Build history of the part. All positions in model axes, mm. A direction names the side the tool comes from. Round coordinates to 2 decimals unless told otherwise and drop trailing zeros. Write each loop counter-clockwise with the first axis right and the second up, starting at its lowest first coordinate (ties: lowest second). Pieces come first, ordered by that corner, then holes. Notation, with made-up numbers: (-12.75, -32.75) -> (8.25, -32.75) arc R21 ccw to (8.25, -25.75) -> close; hole circle Ø3 at (38.25, 39.25). An arc over 180 degrees is marked (long way). Answer in a Markdown table with one row per item. Add a question column.
from build123d import *

# Parameters (mm, degrees)
SKETCH_1_R      = 2.3
EXTRUDE_1_DEPTH = 10
SKETCH_2_W      = 10
SKETCH_2_H      = 15
EXTRUDE_2_DEPTH = 100
SKETCH_3_R      = 2.3
EXTRUDE_3_DEPTH = 10
CHAMFER_1_SIZE  = 5


with BuildPart() as part:
    # Эскиз1 → Бобышка-Вытянуть1 (new body)
    with BuildSketch(Plane(origin=(0, 116.195974268, 0), x_dir=(1, 0, 0), z_dir=(0, 1, 0))):
        Polygon((-8.441019306, -97.523129836), (-8.441019306, -81.523129836), (-8.441019306, -66.523129836), (1.558980694, -66.523129836), (1.558980694, -112.523129836), (-8.441019306, -112.523129836), align=None)
        with Locations(Location((-3.441019306, -89.187817333, 0), (0, 0, 180))):
            Circle(SKETCH_1_R, mode=Mode.SUBTRACT)
    extrude(amount=EXTRUDE_1_DEPTH)

    # Эскиз2 → Бобышка-Вытянуть2 (add)
    with BuildSketch(Plane(origin=(0, 126.195974268, 0), x_dir=(1, 0, 0), z_dir=(0, 1, 0))):
        with Locations((-3.441019306, -74.023129836)):
            Rectangle(SKETCH_2_W, SKETCH_2_H)
        with Locations((-3.441019306, -105.023129836)):
            Rectangle(SKETCH_2_W, SKETCH_2_H)
    extrude(amount=EXTRUDE_2_DEPTH)

    # Эскиз3 → Бобышка-Вытянуть3 (add)
    with BuildSketch(Plane(origin=(0, 226.195974268, 0), x_dir=(1, 0, 0), z_dir=(0, 1, 0))):
        Polygon((-8.441019306, -66.543886748), (-8.441019306, -112.425486731), (1.558980694, -112.523129836), (1.558980694, -66.523129836), align=None)
        with Locations(Location((-3.441019306, -89.187817333, 0), (0, 0, 180))):
            Circle(SKETCH_3_R, mode=Mode.SUBTRACT)
    extrude(amount=EXTRUDE_3_DEPTH)

    # Фаска1
    # the kernel refuses this chamfer: 5 mm, written as the material it takes off along each edge
    with BuildSketch(Plane(origin=(-8.441019306, 239.054389208, 66.523129836), x_dir=(-0.027495876610586625, 0, 0.9996219169112968), z_dir=(0, -1, 0)), Plane(origin=(-8.441019306, 103.337559328, 112.523129836), x_dir=(-0.027495876610585935, 0, -0.9996219169112968), z_dir=(0, 1, 0))) as chamfer_1_piece_1:
        Polygon((CHAMFER_1_SIZE * 0.999621916911, -CHAMFER_1_SIZE * 0.0274958766106), (-CHAMFER_1_SIZE * 0.0274958766106, -CHAMFER_1_SIZE * 0.999621916911), (0, 0), align=None)
    extrude(amount=135.71682988, mode=Mode.SUBTRACT)


solid = part.part
(1) Probe line 1 along Y through (x, z) = (-5.75, 94); line 2 along Z through (x, y) = (-0.75, 154); line 3 along Z through (x, y) = (-3.5, 149). List the from-to ranges inside material, lowest first.
(2) Mould opens along Y. For faces 3 (the face through (-6, 226.196, 89)), 4 (the face through (-5.976, 175.356, 109.988)), 5 (the face through (0, 236.196, 89)) say: pulls with the +Y half, pulls with the -Y half, needs draft (parallel to the pull), parting line crosses it, or undercut.
(3) Saw through at C-C (x = -7). List the corners of the cut face in (y, z).
(4) Saw through at B-B (z = 84). List the corners of the cut face in (x, y).
(5) Saw through at A-A (y = 212). List the corners of the cut face in (x, z).
(6) Drop flat-ended pins along their axis: P1, Ø6, axis at x = -3.44, z = 89.19, coming from the +Y side; P2, Ø10, axis at y = 199, z = 90.5, coming from the -X side; P3, Ø5, axis at x = -7.5, y = 174.5, coming from the -Z side. Give the stop position or say it passes through.
(7) Which spindle directions (+Z, -Z, +X, -X, +Y, -Y) get a long thin tool onto all of the face, cutting with end or side? Do faces 1 (the face through (-5.98, 177.04, 69.06)), 2 (the face through (-4, 175, 81.523)). Say none if no direction does.
Answer sheet:
| question | item | result |
|---|---|---|
| 1 | line 1 | y = 116.2 to 126.2, 226.2 to 236.2 |
| 1 | line 2 | z = 66.52 to 81.52, 97.52 to 112.52 |
| 1 | line 3 | z = 66.58 to 81.52, 97.52 to 112.46 |
| 2 | face 3 | undercut |
| 2 | face 4 | needs draft |
| 2 | face 5 | pulls with the +Y half |
| 3 | outline | (116.2, 70.08) -> (236.2, 70.08) -> (236.2, 108.96) -> (116.2, 108.96) -> close; hole (126.2, 81.52) -> (226.2, 81.52) -> (226.2, 97.52) -> (126.2, 97.52) -> close |
| 4 | outline | (-8.44, 116.2) -> (1.56, 116.2) -> (1.56, 126.2) -> (-8.44, 126.2) -> close; (-8.44, 226.2) -> (1.56, 226.2) -> (1.56, 236.2) -> (-8.44, 236.2) -> close |
| 5 | outline | (-8.44, 71.52) -> (-3.44, 66.52) -> (1.56, 66.52) -> (1.56, 81.52) -> (-8.44, 81.52) -> close; (-8.44, 97.52) -> (1.56, 97.52) -> (1.56, 112.52) -> (-3.44, 112.52) -> (-8.44, 107.52) -> close |
| 6 | P1 | stops at y = 236.2 |
| 6 | P2 | passes through |
| 6 | P3 | stops at z = 68.08 |
| 7 | face 1 | -Z, -X, +Y, -Y |
| 7 | face 2 | +X, -X |
